Geometry check sheet. Reference: the model listing, model coordinates, mm. Coordinates: 2 decimals unless noted, no trailing zeros. Write each loop counter-clockwise with the first axis right and the second up, starting at its lowest first coordinate (ties: lowest second). Pieces come first, ordered by that corner, then holes. Notation, with made-up numbers: M 33,8.25 L 81,8.25 A21 ccw 81,44.25 Z; hole C -8,36 d7. An arc over 180 degrees is marked long. Write item = value, one per line. Start each with the question number.
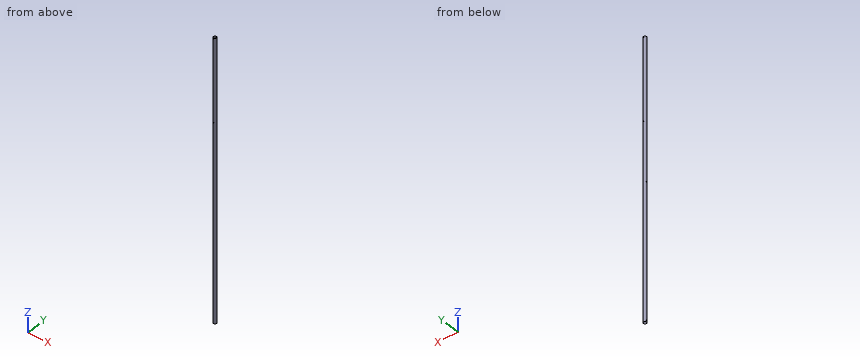
```python
from build123d import *

# Parameters (mm, degrees)
SKETCH1_R               = 12.7
SKETCH1_R_2             = 11.90625
BOSS_EXTRUDE1_DEPTH     = 2443.872227937
SKETCH4_W               = 2.75
SKETCH4_H               = 12.7
SKETCH12_W              = 2.75
SKETCH12_H              = 12.7
SKETCH13_R              = 2.750000003
CUT_EXTRUDE1_DEPTH      = 13.7000001
CUT_EXTRUDE1_DEPTH_BACK = 13.7000001
SKETCH14_R              = 2.5
CUT_EXTRUDE2_DEPTH      = 13.7000001
CUT_EXTRUDE2_DEPTH_BACK = 13.7000001


with BuildPart() as part:
    # Sketch1 → Boss-Extrude1 (new body)
    with BuildSketch(Plane.XY):
        Circle(SKETCH1_R)
        Circle(SKETCH1_R_2, mode=Mode.SUBTRACT)
    extrude(amount=BOSS_EXTRUDE1_DEPTH)

    # Sketch4 → M5 Clearance Hole1 (revolve, cut)
    with BuildSketch(Plane(origin=(0, 0, 2436.622227937), x_dir=(0, 0, -1), z_dir=(1, 0, 0))):
        with Locations((1.375, 6.35)):
            Rectangle(SKETCH4_W, SKETCH4_H)
    m5_clearance_hole1 = revolve(axis=Axis((0, -6.35, 2436.622227937), (0, 1, 0)), mode=Mode.SUBTRACT)

    # Mirror1: M5 Clearance Hole1 across plane
    add(m5_clearance_hole1.mirror(Plane.ZX), mode=Mode.SUBTRACT)

    # Sketch12 → M5 Clearance Hole3 (revolve, cut)
    with BuildSketch(Plane(origin=(0, 0, 15), x_dir=(0, 0, 1), z_dir=(0, 1, 0))):
        with Locations((1.375, 6.35)):
            Rectangle(SKETCH12_W, SKETCH12_H)
    m5_clearance_hole3 = revolve(axis=Axis((-6.35, 0, 15), (1, 0, 0)), mode=Mode.SUBTRACT)

    # Mirror3: M5 Clearance Hole3 across plane
    add(m5_clearance_hole3.mirror(Plane(origin=(0, 0, 0), x_dir=(0, 0, 1), z_dir=(1, 0, 0))), mode=Mode.SUBTRACT)

    # Sketch13 → Cut-Extrude1 (cut, two sides)
    with BuildSketch(Plane(origin=(0, 0, 0), x_dir=(1, 0, 0), z_dir=(0, 1, 0))) as cut_extrude1_sk:
        with Locations((-0.739798723, -1718.754532743)):
            Circle(SKETCH13_R)
    extrude(amount=CUT_EXTRUDE1_DEPTH, mode=Mode.SUBTRACT)
    extrude(cut_extrude1_sk.sketch, amount=-CUT_EXTRUDE1_DEPTH_BACK, mode=Mode.SUBTRACT)

    # Sketch14 → Cut-Extrude2 (cut, two sides)
    with BuildSketch(Plane(origin=(0, 0, 0), x_dir=(0, 0, -1), z_dir=(1, 0, 0))) as cut_extrude2_sk:
        with Locations((-1200, 0)):
            Circle(SKETCH14_R)
    extrude(amount=CUT_EXTRUDE2_DEPTH, mode=Mode.SUBTRACT)
    extrude(cut_extrude2_sk.sketch, amount=-CUT_EXTRUDE2_DEPTH_BACK, mode=Mode.SUBTRACT)


solid = part.part
```
Q1. Gauge pin test, flat ends, axial feed: pin 1 (5 mm diameter, centred on y = 5, z = 474, fed in from -X); pin 2 (4 mm diameter, centred on y = -5.5, z = 848, fed in from -X); pin 3 (1 mm diameter, centred on x = 7.5, z = 520, fed in from +Y). Record the tip position at first contact, or that the pin passes through.
Q2. Cross-section at C-C on z = 958. Enter the section's corners in (x, y).
Q3. Cross-section at B-B on y = -6.75. Enter the section's corners in (x, z).
Q4. Cross-section at A-A on x = -7.75. Enter the section's corners in (y, z), and give its area (3 significant figures).
Q5. Scan lines: L1, parallel to Z at x = 12, y = 0; L2, parallel to Y at x = 4.5, z = 517.5; L3, parallel to Y at x = -1.75, z = 1679.5. Record each from-to range of solid material in increasing order.
Values found:
q1.pin_1 = -12.45
q1.pin_2 = -12.21
q1.pin_3 = 10.6
q2.outline = C 0,0 d25.4; hole C 0,0 d23.81
q3.outline = M -10.76,0 L -9.81,0 L -9.81,2443.87 L -10.76,2443.87 Z; M 9.81,0 L 10.76,0 L 10.76,2443.87 L 9.81,2443.87 Z
q4.outline = M -10.06,0 L -9.04,0 L -9.04,2443.87 L -10.06,2443.87 Z; M 9.04,0 L 10.06,0 L 10.06,2443.87 L 9.04,2443.87 Z
q4.area = 5,000 mm²
q5.L1 = 0 to 12.25, 17.75 to 1197.5, 1202.5 to 2443.87
q5.L2 = -11.88 to -11.02, 11.02 to 11.88
q5.L3 = -12.58 to -11.78, 11.78 to 12.58
